Part print with two shaded views. Sizes in mm from the minimum x, y, z corner. A direction names the side the tool comes from. Coordinates: 2 decimals unless noted, no trailing zeros. Loops run counter-clockwise (first coordinate to the right, second up) from the corner with the lowest first, then second, coordinate; pieces in that order, holes last.
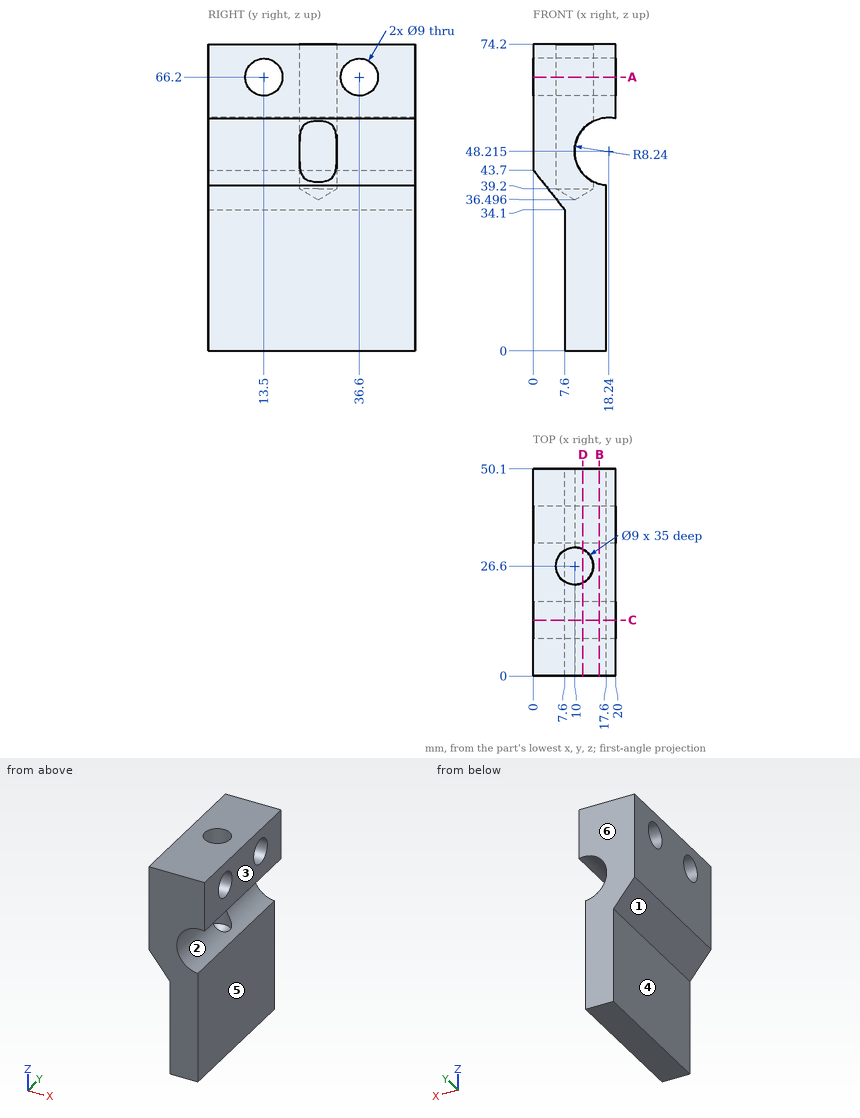
Q1. Slice it at D-D (x = 12). Count the separate pieces of the cut face and the enclosed holes in it, and give its area (3 significant figures).
Answers:
separate pieces: 3
enclosed holes: 2
area: 2,850 mm2
Q2. Flat gauge pins, fed straight in: P1, Ø3, axis at y = 21, z = 19, coming from the -X side; P2, Ø2, axis at y = 12, z = 33.5, coming from the +X side; P3, Ø8, axis at y = 36.6, z = 66.2, coming from the -X side; P4, Ø4, axis at y = 22, z = 52, coming from the +X side. Where does each tip first touch, or does it go through?
Answers:
P1: stops at x = 7.6
P2: stops at x = 17.6
P3: passes through
P4: stops at x = 12.37
Q3. Slice it at A-A (z = 66.2). List the corners of the cut face in (x, y), and give its area (3 significant figures).
Answers:
outline: (0, 0) - (20, 0) - (20, 9) - (0, 9) - close; (0, 18) - (20, 18) - (20, 32.1) - (0, 32.1) - close; (0, 41.1) - (20, 41.1) - (20, 50.1) - (0, 50.1) - close; hole circle Ø9 at (10, 26.6)
area: 578 mm2
Q4. Slice it at C-C (y = 13.5). List the corners of the cut face in (x, z) (1 decimal), and give its area (3 significant figures).
Answers:
outline: (0, 43.7) - (7.6, 34.1) - (7.6, 0) - (17.6, 0) - (17.6, 40) arc R8.2 cw (long way) to (20, 56.3) - (20, 61.7) - (0, 61.7) - close; (0, 70.7) - (20, 70.7) - (20, 74.2) - (0, 74.2) - close
area: 777 mm2
Q5. Slice it at B-B (x = 16). List the corners of the cut face in (y, z).
Answers:
outline: (0, 0) - (50.1, 0) - (50.1, 40.29) - (0, 40.29) - close; (0, 56.14) - (50.1, 56.14) - (50.1, 74.2) - (0, 74.2) - close; hole circle Ø9 at (13.5, 66.2); hole circle Ø9 at (36.6, 66.2)
Q6. Mould opens along Z. For the marked faces 1, 2 and 3 say: +Z half, -Z half, draft (parallel to the pull), parting line (faces both ways), or undercut.
Answers:
face 1: -Z half
face 2: undercut
face 3: draft
Q7. Which spindle directions (+Z, -Z, +X, -X, +Y, -Y) get a long thin tool onto all of the face, cutting with end or side? Do the marked faces 4, 5 and 6. Say none if no direction does.
Answers:
face 4: -Z, -X, +Y, -Y
face 5: -Z, +X, +Y, -Y
face 6: +Z, -Z, +X, -X, +Y
Q8. Drill centre lines: line 1 (Y direction, x = 10, z = 47.5); line 2 (Z direction, x = 8.25, y = 36.6); line 3 (Z direction, x = 15.75, y = 15). Where is each one in solid material? Low to high.
Answers:
line 1: y = 0 to 22.1, 31.1 to 50.1
line 2: z = 0 to 61.7, 70.7 to 74.2
line 3: z = 0 to 40.36, 56.07 to 61.96, 70.44 to 74.2
